from build123d import *

# Parameters (mm, degrees)
SKETCH_1_W          = 25
SKETCH_1_H          = 30
EXTRUDE_1_DEPTH     = 2
SKETCH_2_W          = 20.6
SKETCH_2_H          = 25.6
EXTRUDE_2_DEPTH     = 5
SKETCH_3_W          = 16.6
SKETCH_3_H          = 21.6
CUT_EXTRUDE_1_DEPTH = 5
SKETCH_4_W          = 6.2
SKETCH_4_H          = 6.2
CUT_EXTRUDE_2_DEPTH = 1
SKETCH_5_R          = 6.05
CUT_EXTRUDE_3_DEPTH = 1


with BuildPart() as part:
    # ｽｹｯﾁ1 → ﾎﾞｽ - 押し出し1 (new body)
    with BuildSketch(Plane.XY):
        with Locations((-24.237274581, 24.707142857)):
            Rectangle(SKETCH_1_W, SKETCH_1_H)
    extrude(amount=EXTRUDE_1_DEPTH)

    # ｽｹｯﾁ2 → ﾎﾞｽ - 押し出し2 (add)
    with BuildSketch(Plane.XY.offset(2)):
        with Locations((-24.237274581, 24.707142857)):
            Rectangle(SKETCH_2_W, SKETCH_2_H)
    extrude(amount=EXTRUDE_2_DEPTH)

    # ｽｹｯﾁ3 → ｶｯﾄ - 押し出し1 (cut)
    with BuildSketch(Plane.XY.offset(7)):
        with Locations((-24.237274581, 24.707142857)):
            Rectangle(SKETCH_3_W, SKETCH_3_H)
    extrude(amount=-CUT_EXTRUDE_1_DEPTH, mode=Mode.SUBTRACT)

    # ｽｹｯﾁ4 → ｶｯﾄ - 押し出し2 (cut)
    with BuildSketch(Plane(origin=(0, 0, 0), x_dir=(-1, 0, 0), z_dir=(0, 0, -1))):
        with Locations((14.837274581, 36.607142857)):
            Rectangle(SKETCH_4_W, SKETCH_4_H)
        with Locations((33.637274581, 36.607142857)):
            Rectangle(SKETCH_4_W, SKETCH_4_H)
        with Locations((33.637274581, 17.807142857)):
            Rectangle(SKETCH_4_W, SKETCH_4_H)
        with Locations((14.837274581, 17.807142857)):
            Rectangle(SKETCH_4_W, SKETCH_4_H)
    extrude(amount=-CUT_EXTRUDE_2_DEPTH, mode=Mode.SUBTRACT)

    # ｽｹｯﾁ5 → ｶｯﾄ - 押し出し3 (cut)
    with BuildSketch(Plane.XY.offset(2)):
        with Locations((-24.237274581, 24.707142857)):
            Circle(SKETCH_5_R)
    extrude(amount=-CUT_EXTRUDE_3_DEPTH, mode=Mode.SUBTRACT)


solid = part.part
Part model, mm, in its own coordinate system. A direction names the side the tool comes from. Give positions to 0.01 mm unless a question says otherwise; leave off trailing zeros. Order: outer loops, then holes, each group sorted by start corner. A loop starts at its lowest first (then second) coordinate and runs counter-clockwise, first axis right, second up. Notation, with made-up numbers: (-26.75, 50.25) -> (0.25, 50.25) arc R22 cw to (0.25, 76.25) -> close; hole circle Ø4 at (78, 74). An arc over 180 degrees is marked (long way). Use one line per item in the form item = value.
(1) Tool access for faces 1 (the face through (-34.537, 25, 4)), 2 (the face through (-24, 11.907, 4)), 3 (the face through (-30.537, 17.8, 0.5)): list every direction of +Z, -Z, +X, -X, +Y, -Y with a clear straight run to the whole face (end or side of a thin tool).
Solution:
face_1 = +Z, -X, +Y, -Y
face_2 = +Z, +X, -X, -Y
face_3 = -Z, -X
(2) Saw through at B-B (z = 4.25). Write the cut outline in (x, y).
Solution:
outline = (-34.54, 11.91) -> (-13.94, 11.91) -> (-13.94, 37.51) -> (-34.54, 37.51) -> close; hole (-32.54, 13.91) -> (-15.94, 13.91) -> (-15.94, 35.51) -> (-32.54, 35.51) -> close
(3) Saw through at A-A (y = 38). Write the cut outline in (x, z), then the cut area to 3 significant figures.
Solution:
outline = (-36.74, 1) -> (-30.54, 1) -> (-30.54, 0) -> (-17.94, 0) -> (-17.94, 1) -> (-11.74, 1) -> (-11.74, 2) -> (-36.74, 2) -> close
area = 37.6 mm²
(4) Saw through at C-C (x = -14.5). Write the cut outline in (y, z), then the cut area to 3 significant figures.
Solution:
outline = (9.71, 0) -> (14.71, 0) -> (14.71, 1) -> (20.91, 1) -> (20.91, 0) -> (33.51, 0) -> (33.51, 1) -> (39.71, 1) -> (39.71, 2) -> (37.51, 2) -> (37.51, 7) -> (11.91, 7) -> (11.91, 2) -> (9.71, 2) -> close
area = 176 mm²
(5) Drill centre lines: line 1 (X direction, y = 23.25, z = 3.5); line 2 (Y direction, x = -24.5, z = 3.5); line 3 (Z direction, x = -12.75, y = 19.75). Where is each one in solid material? Low to high. Write a range as from..to.
Solution:
line_1 = -34.54..-32.54, -15.94..-13.94
line_2 = 11.91..13.91, 35.51..37.51
line_3 = 1..2
(6) Saw through at D-D (y = 14.25). Write the cut outline in (x, z).
Solution:
outline = (-36.74, 0) -> (-11.74, 0) -> (-11.74, 2) -> (-13.94, 2) -> (-13.94, 7) -> (-15.94, 7) -> (-15.94, 2) -> (-32.54, 2) -> (-32.54, 7) -> (-34.54, 7) -> (-34.54, 2) -> (-36.74, 2) -> close
(7) Flat gauge pins, fed straight in: P1, Ø0.8, axis at x = -32.5, z = 0.5, coming from the +Y side; P2, Ø10, axis at x = -23.5, y = 29, coming from the +Z side; P3, Ø1.9, axis at x = -35, y = 37.5, coming from the -Z side. Where does each tip first touch, or does it go through?
Solution:
P1 = 33.51
P2 = 2
P3 = 1
(8) Pull direction X, two halves, no side cores. Call faces 4 (the face through (-34, 18, 1)), 5 (the face through (-32.537, 25, 5)), 6 (the face through (-11.737, 24, 1)), 7 (the face through (-15.937, 25, 5)): +X half, -X half, draft (parallel to the pull), parting line (faces both ways), or undercut.
Solution:
face_4 = draft
face_5 = undercut
face_6 = +X half
face_7 = undercut
